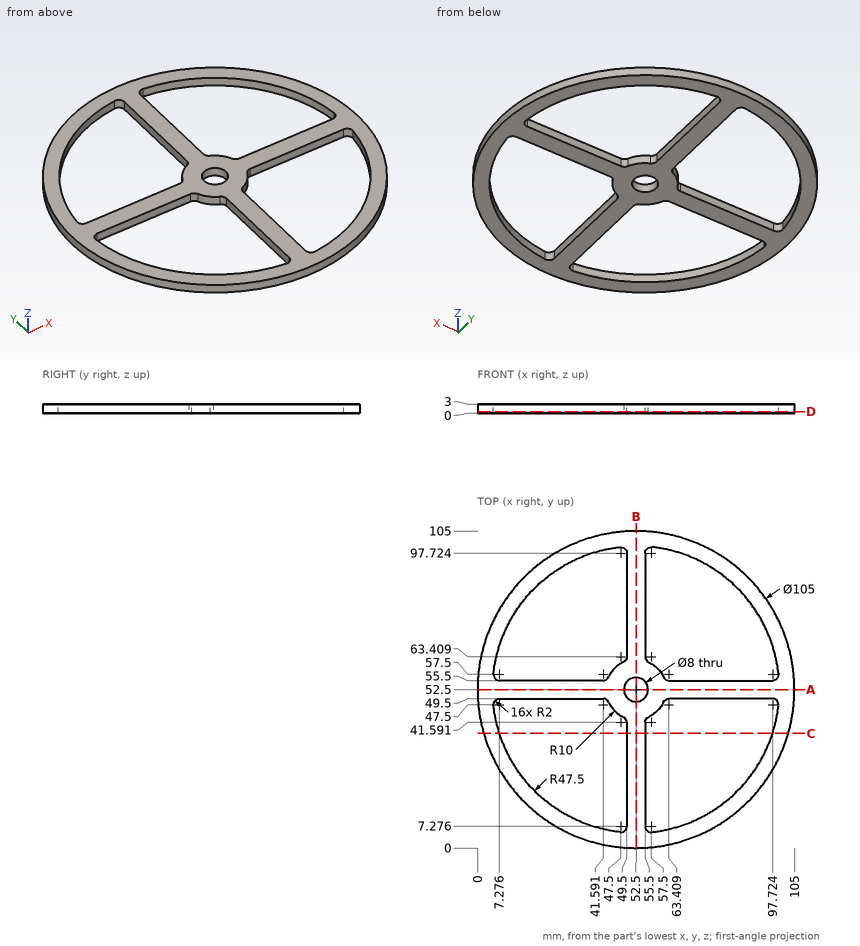
Here's the drawing with two shaded views (mm, measured from the low corner). I have some questions. Round coordinates to 2 decimals unless told otherwise and drop trailing zeros. Loops run counter-clockwise (first coordinate to the right, second up) from the corner with the lowest first, then second, coordinate; pieces in that order, holes last. Notation, with made-up numbers: (52.5, -14) - (85.5, -14) arc R6 ccw to (85.5, -6) - close; hole circle Ø4 at (65, 37.25). An arc over 180 degrees is marked (long way). Write item = value, one per line.
1) I'm going to push flat-ended pins straight in: P1, Ø0.9, axis at x = 17, z = 2, coming from the -Y side (1 decimal); P2, Ø2, axis at x = 52.5, y = 69.5, coming from the -Z side; P3, Ø1.5, axis at y = 28.5, z = 1, coming from the +X side; P4, Ø1.5, axis at x = 81, z = 1, coming from the +Y side. Where does each tip first touch, or does it pass through?
Computed:
P1 = 13.4
P2 = 0
P3 = 99.57
P4 = 97.07
2) I need wall thicknesses on line 1 along X through (y, z) = (35.5, 0.8) (1 decimal); line 2 along X through (y, z) = (60.5, 1.3) (1 decimal); line 3 along Y through (x, z) = (27, 1.15) (1 decimal). Which ranges of each line are inside material? Lowest first, please. Write a range as from..to.
Computed:
line_1 = 2.8..8.1, 49.5..55.5, 96.9..102.2
line_2 = 0.6..5.7, 46.5..58.5, 99.3..104.4
line_3 = 6.6..12.4, 49.5..55.5, 92.6..98.4
3) Imagine slicing it at D-D (z = 0.5). Give the number of separate pieces and of enclosed holes in the cut face, and give its area (3 significant figures).
Computed:
separate_pieces = 1
enclosed_holes = 5
area = 2,750 mm2
4) Imagine slicing it at C-C (y = 38). Please give me the cut outline in (x, z).
Computed:
outline = (2.04, 0) - (7.27, 0) - (7.27, 3) - (2.04, 3) - close; (49.5, 0) - (55.5, 0) - (55.5, 3) - (49.5, 3) - close; (97.73, 0) - (102.96, 0) - (102.96, 3) - (97.73, 3) - close
5) Imagine slicing it at A-A (y = 52.5). Please give me the cut outline in (x, z).
Computed:
outline = (0, 0) - (48.5, 0) - (48.5, 3) - (0, 3) - close; (56.5, 0) - (105, 0) - (105, 3) - (56.5, 3) - close
